Geometry: final body of the model. Coordinates: model frame, mm. Face numbers are marked on the shaded views. A direction names the side the tool comes from. Round coordinates to 2 decimals unless told otherwise and drop trailing zeros. Write each loop counter-clockwise with the first axis right and the second up, starting at its lowest first coordinate (ties: lowest second). Pieces come first, ordered by that corner, then holes. Notation, with made-up numbers: (-0.5, -27.75) -> (3.5, -27.75) arc R20 ccw to (3.5, 8.25) -> close; hole circle Ø1 at (-40, 49.5). An arc over 180 degrees is marked (long way). Use one line per item in the form item = value. Start each with the question number.
1. Cut plane C-C, the plane z = 40.5. Return the cut outline in (x, y).
2. Line query: L1, parallel to X at y = 1.6, z = 52.5; L2, parallel to X at y = 1.25, z = 50.5; L3, parallel to Y at x = -49.5, z = -56. Output: solid intervals per line, ascending.
3. Cut plane B-B, the plane z = -52.5. Return the cut outline in (x, y).
4. Cut plane D-D, the plane x = 15. Return the cut outline in (y, z), plus the area to 3 significant figures.
5. Reachability of the marked faces 1 and 2 from +Z, -Z, +X, -X, +Y, -Y: full face, straight path, thin tool, end or side. Return the list, or none.
6. Cut plane A-A, the plane x = -52.5. Return the cut outline in (y, z), plus the area to 3 significant figures.
7. Pin query (flat end, axial travel): pin 1 Ø0.8 at (x, y) = (55, 2.5) entering from -Z; pin 2 Ø4 at (x, z) = (52.5, -52.5) entering from -Y; pin 3 Ø0.5 at (x, y) = (49.5, 2.5) entering from +Z. Return the tip coordinate at first contact, or that it passes through.
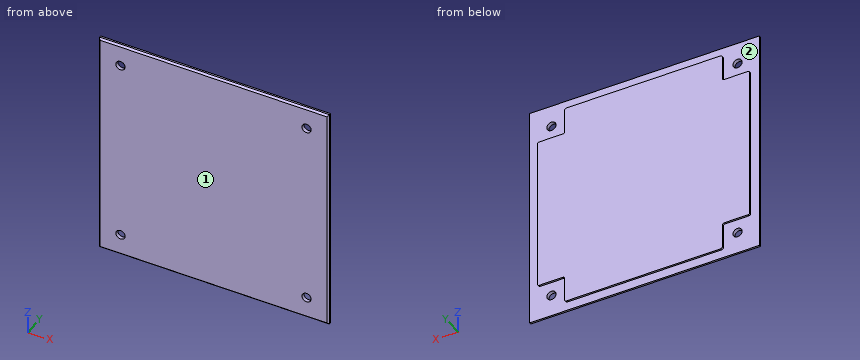
```python
from build123d import *

# Parameters (mm, degrees)
SKETCH_1_W          = 130
SKETCH_1_H          = 130
EXTRUDE_1_DEPTH     = 3
SKETCH_2_R          = 2.6
CUT_EXTRUDE_1_DEPTH = 92.972822073
SKETCH_4_W          = 20.5
SKETCH_4_H          = 20.5
CUT_EXTRUDE_2_DEPTH = 1
SKETCH_5_W          = 89
SKETCH_5_H          = 5.1
SKETCH_5_W_2        = 5.1
SKETCH_5_H_2        = 89
CUT_EXTRUDE_3_DEPTH = 1
CHAMFER_1_SIZE      = 0.2
CHAMFER_2_SIZE      = 1
FILLET_2_R          = 1


with BuildPart() as part:
    # 草图1 → 凸台-拉伸1 (new body)
    with BuildSketch(Plane(origin=(0, 0, 0), x_dir=(1, 0, 0), z_dir=(0, 1, 0))):
        Rectangle(SKETCH_1_W, SKETCH_1_H)
    extrude(amount=EXTRUDE_1_DEPTH)

    # 草图2 → 切除-拉伸1 (cut, through all)
    with BuildSketch(Plane(origin=(0, 3, 0), x_dir=(1, 0, 0), z_dir=(0, 1, 0))):
        with Locations(Location((52.5, 52.5, 0), (0, 0, 270))):
            Circle(SKETCH_2_R)
        with Locations(Location((52.5, -52.5, 0), (0, 0, 270))):
            Circle(SKETCH_2_R)
        with Locations(Location((-52.5, -52.5, 0), (0, 0, 270))):
            Circle(SKETCH_2_R)
        with Locations(Location((-52.5, 52.5, 0), (0, 0, 270))):
            Circle(SKETCH_2_R)
    extrude(amount=-CUT_EXTRUDE_1_DEPTH, mode=Mode.SUBTRACT)

    # 草图4 → 切除-拉伸2 (cut)
    with BuildSketch(Plane(origin=(0, 3, 0), x_dir=(1, 0, 0), z_dir=(0, 1, 0))):
        with Locations((54.75, 54.75)):
            Rectangle(SKETCH_4_W, SKETCH_4_H)
        with Locations((54.75, -54.75)):
            Rectangle(SKETCH_4_W, SKETCH_4_H)
        with Locations((-54.75, -54.75)):
            Rectangle(SKETCH_4_W, SKETCH_4_H)
        with Locations((-54.75, 54.75)):
            Rectangle(SKETCH_4_W, SKETCH_4_H)
    extrude(amount=-CUT_EXTRUDE_2_DEPTH, mode=Mode.SUBTRACT)

    # 草图5 → 切除-拉伸3 (cut)
    with BuildSketch(Plane(origin=(0, 3, 0), x_dir=(1, 0, 0), z_dir=(0, 1, 0))):
        with Locations((0, 62.45)):
            Rectangle(SKETCH_5_W, SKETCH_5_H)
        with Locations((62.45, 0)):
            Rectangle(SKETCH_5_W_2, SKETCH_5_H_2)
        with Locations((0, -62.45)):
            Rectangle(SKETCH_5_W, SKETCH_5_H)
        with Locations((-62.45, 0)):
            Rectangle(SKETCH_5_W_2, SKETCH_5_H_2)
    extrude(amount=-CUT_EXTRUDE_3_DEPTH, mode=Mode.SUBTRACT)

    # 倒角1
    chamfer_1_edges = [part.edges().sort_by_distance(p)[0] for p in [
        (65, 1, 65),
        (-65, 1, 65),
        (-65, 1, -65),
        (65, 1, -65),
    ]]
    chamfer(chamfer_1_edges, length=CHAMFER_1_SIZE)

    # 倒角2
    # the kernel refuses this chamfer: 1 mm, written as the material it takes off along each edge
    with BuildSketch(Plane(origin=(67.371682988, 0, 65), x_dir=(0, -0.027495876610586292, -0.9996219169112968), z_dir=(-1, 0, 0)), Plane(origin=(65, 0, -67.371682988), x_dir=(-0.9996219169112968, -0.027495876610586292, 0), z_dir=(0, 0, 1)), Plane(origin=(-65, 0, 67.371682988), x_dir=(0.9996219169112968, -0.027495876610586292, 0), z_dir=(0, 0, -1))) as chamfer_2_piece_1:
        Polygon((CHAMFER_2_SIZE * 0.999621916911, -CHAMFER_2_SIZE * 0.0274958766106), (-CHAMFER_2_SIZE * 0.0274958766106, -CHAMFER_2_SIZE * 0.999621916911), (0, 0), align=None)
    extrude(amount=134.743365976, mode=Mode.SUBTRACT)
    with BuildSketch(Plane(origin=(-67.371682988, 0, -65), x_dir=(0, 0.999621916911297, -0.02749587661058218), z_dir=(1, 0, 0))) as chamfer_2_piece_2:
        Polygon((CHAMFER_2_SIZE * 0.999621916911, CHAMFER_2_SIZE * 0.0274958766106), (-CHAMFER_2_SIZE * 0.0274958766106, CHAMFER_2_SIZE * 0.999621916911), (0, 0), align=None)
    extrude(amount=134.743365976, mode=Mode.SUBTRACT)

    # 圆角2
    fillet_2_edges = [part.edges().sort_by_distance(p)[0] for p in [
        (-44.5, 2.5, -59.9),
        (44.5, 2.5, -59.9),
        (59.9, 2.5, -44.5),
        (59.9, 2.5, 44.5),
        (44.5, 2.5, 59.9),
        (-44.5, 2.5, 59.9),
        (-59.9, 2.5, 44.5),
        (-59.9, 2.5, -44.5),
        (-44.5, 2.5, -44.5),
        (-44.5, 2.5, 44.5),
        (44.5, 2.5, 44.5),
        (44.5, 2.5, -44.5),
    ]]
    fillet(fillet_2_edges, radius=FILLET_2_R)


solid = part.part
```
Outcome:
q1.outline = (-65, 1) -> (-64, 0) -> (64, 0) -> (65, 1) -> (65, 2) -> (59.9, 2) -> (59.9, 3) -> (-59.9, 3) -> (-59.9, 2) -> (-65, 2) -> close
q2.L1 = -65 to -55.1, -49.9 to 49.9, 55.1 to 65
q2.L2 = -65 to -54.16, -50.84 to 50.84, 54.16 to 65
q2.L3 = 0 to 2
q3.outline = (-65, 1) -> (-64, 0) -> (-55.1, 0) -> (-55.1, 2) -> (-65, 2) -> close; (-49.9, 0) -> (49.9, 0) -> (49.9, 2) -> (44.5, 2) -> (44.5, 3) -> (-44.5, 3) -> (-44.5, 2) -> (-49.9, 2) -> close; (55.1, 0) -> (64, 0) -> (65, 1) -> (65, 2) -> (55.1, 2) -> close
q4.outline = (0, -64) -> (1, -65) -> (2, -65) -> (2, -59.9) -> (3, -59.9) -> (3, 59.9) -> (2, 59.9) -> (2, 65) -> (1, 65) -> (0, 64) -> close
q4.area = 379 mm^2
q5.face_1 = +Z, -Z, +X, -X, -Y
q5.face_2 = +Y
q6.outline = (0, -64) -> (1, -65) -> (2, -65) -> (2, -55.1) -> (0, -55.1) -> close; (0, -49.9) -> (2, -49.9) -> (2, -44.5) -> (3, -44.5) -> (3, 44.5) -> (2, 44.5) -> (2, 49.9) -> (0, 49.9) -> close; (0, 55.1) -> (2, 55.1) -> (2, 65) -> (1, 65) -> (0, 64) -> close
q6.area = 327 mm^2
q7.pin_1 = -44.5
q7.pin_2 = through
q7.pin_3 = 44.5
